Check sheet for the modelled part. Datum: model origin and axes. Units: mm. Face numbers are marked on the shaded views. A direction names the side the tool comes from. Round coordinates to 2 decimals unless told otherwise and drop trailing zeros. Write each loop counter-clockwise with the first axis right and the second up, starting at its lowest first coordinate (ties: lowest second). Pieces come first, ordered by that corner, then holes.
Item 1: Material ranges on line 1 along Z through (x, y) = (58, 0.25); line 2 along X through (y, z) = (-2.5, -6); line 3 along X through (y, z) = (-7, -4.25), recorded low to high.
Item 2: Depth check by flat-ended pin: pin 1 (4 mm diameter, centred on y = -7.5, z = 3.5, fed in from +X); pin 2 (8 mm diameter, centred on x = 150.5, z = 0.5, fed in from -Y); pin 3 (2 mm diameter, centred on x = 24.5, y = -9, fed in from -Z). Enter the tip coordinate at first touch or a pass-through.
Item 3: Section check C-C, the plane x = 52.5. Record the cut outline in (y, z).
Item 4: Set-up check for the marked faces 1, 2 and 3: record each of +Z, -Z, +X, -X, +Y, -Y from which the full face is reachable in a straight line by a thin tool's end or side.
Item 5: Section check D-D, the plane x = 96.5. Record the cut outline in (y, z).
Item 6: Section check A-A, the plane y = 0. Record the cut outline in (x, z), plus the area to 3 significant figures.
Autodesk Inventor part; units mm, degrees
ref_plane "YZ Plane" through (0, 0, 0) normal (1, 0, 0) x (0, 1, 0)
ref_plane "XZ Plane" through (0, 0, 0) normal (0, 1, 0) x (-1, 0, 0)
ref_plane "XY Plane" through (0, 0, 0) normal (0, 0, 1) x (1, 0, 0)
sketch "Sketch1" plane through (0, 0, 0) normal (0, 0, 1) x (1, 0, 0)
  line L0 (0, 0) -> (170, 0)
  line L1 (170, 0) -> (170, 5)
  line L2 (170, 5) -> (150, 5)
  line L3 (150, 5) -> (150, 7)
  line L4 (150, 7) -> (90, 7)
  line L5 (90, 7) -> (60, 7)
  line L6 (60, 7) -> (60, 9)
  line L7 (60, 9) -> (28, 9)
  line L8 (28, 9) -> (28, 15)
  line L9 (28, 15) -> (24, 15)
  line L10 (24, 15) -> (24, 11)
  line L11 (24, 11) -> (0, 11)
  line L12 (0, 11) -> (0, 0)
  dimension "d0" = 170
  dimension "d1" = 10
  dimension "d2" = 14
  dimension "d3" = 18
  dimension "d4" = 30
  dimension "d5" = 22
  dimension "d6" = 24
  dimension "d7" = 4
  dimension "d8" = 32
  dimension "d9" = 60
  dimension "d10" = 30
revolve "Revolution1" add sketch "Sketch1" angle 360 about axis through (0, 0, 0) along (1, 0, 0)
thread "Thread1"
fillet "Fillet1" radius 3 1 edges at (28, -9, 0)
fillet "Fillet2" radius 2 1 edges at (0, -11, 0)
chamfer "Chamfer1" distance 1 angle 45 1 edges at (170, -5, 0)
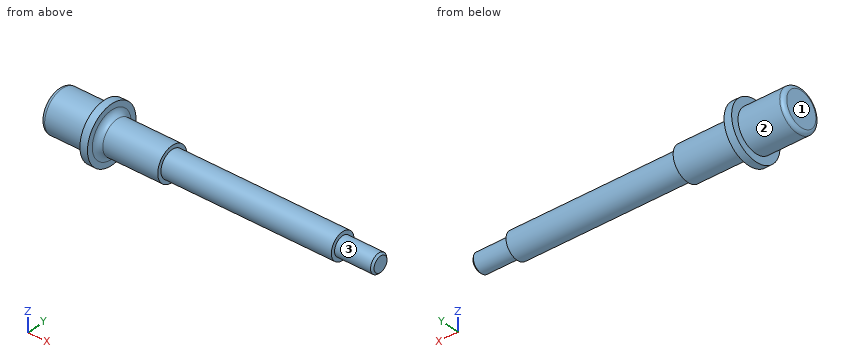
Values found:
1. line 1: z = -9 to 9
1. line 2: x = 0 to 150
1. line 3: x = 0 to 60
2. pin 1: stops at x = 150
2. pin 2: stops at y = -7
2. pin 3: stops at z = -12.69
3. outline: circle Ø18 at (0, 0)
4. face 1: +Z, -Z, -X, +Y, -Y
4. face 2: -X
4. face 3: +X
5. outline: circle Ø14 at (0, 0)
6. outline: (0, -9) arc R2 ccw to (2, -11) - (24, -11) - (24, -15) - (28, -15) - (28, -12) arc R3 cw to (31, -9) - (60, -9) - (60, -7) - (150, -7) - (150, -5) - (169, -5) - (170, -4) - (170, 4) - (169, 5) - (150, 5) - (150, 7) - (60, 7) - (60, 9) - (31, 9) arc R3 cw to (28, 12) - (28, 15) - (24, 15) - (24, 11) - (2, 11) arc R2 ccw to (0, 9) - close
6. area: 2,690 mm2
